Could you check a few things on this model? Use its own coordinates, in mm. Face numbers are marked on the shaded views. A direction names the side the tool comes from. Coordinates: 2 decimals unless noted, no trailing zeros. Write each loop counter-clockwise with the first axis right and the second up, starting at its lowest first coordinate (ties: lowest second). Pieces come first, ordered by that corner, then holes.
```python
from build123d import *

# Parameters (mm, degrees)
SKETCH1_W           = 32
SKETCH1_H           = 7.6
BOSS_EXTRUDE1_DEPTH = 1
SKETCH2_R           = 1
CUT_EXTRUDE1_DEPTH  = 17.475436261
SKETCH3_W           = 1.6
SKETCH3_H           = 2.2
BOSS_EXTRUDE2_DEPTH = 1
SKETCH4_W           = 12.7
SKETCH4_H           = 2.54
BOSS_EXTRUDE3_DEPTH = 11
SKETCH5_W           = 12.7
SKETCH5_H           = 2.54
BOSS_EXTRUDE4_DEPTH = 2.5


with BuildPart() as part:
    # Sketch1 → Boss-Extrude1 (new body)
    with BuildSketch(Plane(origin=(0, 0, 0), x_dir=(1, 0, 0), z_dir=(0, 1, 0))):
        Rectangle(SKETCH1_W, SKETCH1_H)
    extrude(amount=BOSS_EXTRUDE1_DEPTH)

    # Sketch2 → Cut-Extrude1 (cut, through all)
    with BuildSketch(Plane(origin=(0, 1, 0), x_dir=(1, 0, 0), z_dir=(0, 1, 0))):
        with Locations(Location((-13.4, 0, 0), (0, 0, 270))):
            Circle(SKETCH2_R)
        with Locations(Location((13.4, 0, 0), (0, 0, 270))):
            Circle(SKETCH2_R)
    extrude(amount=-CUT_EXTRUDE1_DEPTH, mode=Mode.SUBTRACT)

    # Sketch3 → Boss-Extrude2 (add)
    with BuildSketch(Plane.XZ):
        with Locations((-9.5, 0)):
            Rectangle(SKETCH3_W, SKETCH3_H)
        with Locations((9.5, 0)):
            Rectangle(SKETCH3_W, SKETCH3_H)
        with Locations((0, 1.1)):
            Rectangle(SKETCH3_W, SKETCH3_H)
    extrude(amount=BOSS_EXTRUDE2_DEPTH)

    # Sketch4 → Boss-Extrude3 (add)
    with BuildSketch(Plane(origin=(0, 0, -3.8), x_dir=(-1, 0, 0), z_dir=(0, 0, -1))):
        with Locations((0, -0.17)):
            Rectangle(SKETCH4_W, SKETCH4_H)
    extrude(amount=BOSS_EXTRUDE3_DEPTH)

    # Sketch5 → Boss-Extrude4 (add)
    with BuildSketch(Plane(origin=(0, 1, 0), x_dir=(1, 0, 0), z_dir=(0, 1, 0))):
        with Locations((0, 2.43)):
            Rectangle(SKETCH5_W, SKETCH5_H)
    extrude(amount=BOSS_EXTRUDE4_DEPTH)


solid = part.part
```
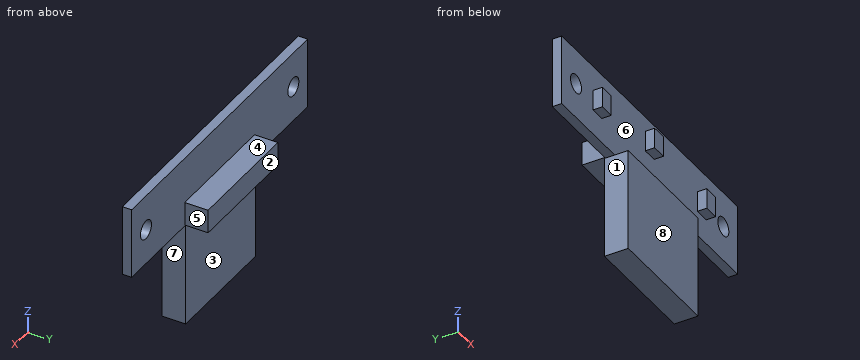
1. For pin 1 (8.5 mm diameter, centred on x = 0, z = 1.5, fed in from -Y); pin 2 (0.5 mm diameter, centred on y = -0.5, z = 0.5, fed in from -X); pin 3 (0.5 mm diameter, centred on x = 9.5, y = -0.5, fed in from +Z), each with a flat end and sliding along its axis, tell me the tip position at first contact or that it passes through.
Verdict:
pin 1: stops at y = -1
pin 2: stops at x = -10.3
pin 3: stops at z = 1.1
2. I want a section at A-A on y = 0.3. Please give me the cut outline in (x, z), plus the area to 3 significant figures.
Verdict:
outline: (-16, -3.8) - (-6.35, -3.8) - (-6.35, -14.8) - (6.35, -14.8) - (6.35, -3.8) - (16, -3.8) - (16, 3.8) - (-16, 3.8) - close; hole circle Ø2 at (-13.4, 0); hole circle Ø2 at (13.4, 0)
area: 377 mm2
3. If we mould it in two halves opening along X, with no side actions, what happens to the marked faces 6, 7 and 8? For each: pulls with the +X half, pulls with the -X half, needs draft (parallel to the pull), parting line crosses it, or undercut.
Verdict:
face 6: undercut
face 7: pulls with the +X half
face 8: needs draft
4. I want a section at B-B on x = 13.4. Please give me the cut outline in (y, z), plus the area to 3 significant figures.
Verdict:
outline: (0, -3.8) - (1, -3.8) - (1, -1) - (0, -1) - close; (0, 1) - (1, 1) - (1, 3.8) - (0, 3.8) - close
area: 5.60 mm2
5. I want a section at C-C on x = -3.5. Please give me the cut outline in (y, z), plus the area to 3 significant figures.
Verdict:
outline: (-1.44, -14.8) - (1.1, -14.8) - (1.1, -3.8) - (1, -3.8) - (1, -3.7) - (3.5, -3.7) - (3.5, -1.16) - (1, -1.16) - (1, 3.8) - (0, 3.8) - (0, -3.8) - (-1.44, -3.8) - close
area: 41.9 mm2
6. On a 3-axis mill with a long thin cutter (end or side, diameter ignored), from which of +Z, -Z, +X, -X, +Y, -Y can I reach the whole of each face in a straight line? I mean the marked faces 1, 2, 3, 4 and 5. Say none if no direction works.
Verdict:
face 1: -Z, -X, +Y, -Y
face 2: +Z, -Z, +X, -X, +Y
face 3: -Z, +X, -X, +Y
face 4: +Z, +X, -X, +Y
face 5: +Z, -Z, +X, +Y
7. I want a section at D-D on z = -10. Please give me the cut outline in (x, y), plus the area to 3 significant figures.
Verdict:
outline: (-6.35, -1.44) - (6.35, -1.44) - (6.35, 1.1) - (-6.35, 1.1) - close
area: 32.3 mm2
8. Please list where these lines run through material, in increasing order: line 1 along X through (y, z) = (0.4, 0); line 2 along X through (y, z) = (0, -10.75); line 3 along Y through (x, z) = (12, -2.75).
Verdict:
line 1: x = -16 to -14.4, -12.4 to 12.4, 14.4 to 16
line 2: x = -6.35 to 6.35
line 3: y = 0 to 1
